```python
from build123d import *

# Parameters (mm, degrees)
SKETCH1_W                 = 180
SKETCH1_H                 = 100
BOSS_EXTRUDE1_DEPTH       = 60
F_3_0MM_DOWEL_HOLE1_D     = 5.25
F_3_0MM_DOWEL_HOLE1_DEPTH = 50
F_3_0MM_DOWEL_HOLE1_TIP   = 1.577259125
SHELL2_START              = 3
SHELL2_DEPTH              = 57
SHELL2_2_DEPTH            = 5.302681665
FILLET1_R                 = 5
FILLET2_R                 = 3
SKETCH4_R                 = 5.959707521
SKETCH4_W                 = 8
SKETCH4_H                 = 15
CUT_EXTRUDE1_DEPTH        = 10
SKETCH6_R                 = 5.5
CUT_EXTRUDE2_DEPTH        = 10
SKETCH9_R                 = 3.5
SKETCH9_R_2               = 5
SKETCH9_R_3               = 4
CUT_EXTRUDE3_DEPTH        = 7
SKETCH10_R                = 4
CUT_EXTRUDE4_DEPTH        = 10


with BuildPart() as part:
    # Sketch1 → Boss-Extrude1 (new body)
    with BuildSketch(Plane(origin=(0, 0, 0), x_dir=(1, 0, 0), z_dir=(0, 1, 0))):
        with Locations((90, -50)):
            Rectangle(SKETCH1_W, SKETCH1_H)
    extrude(amount=BOSS_EXTRUDE1_DEPTH)

    # Ø3.0mm Dowel Hole1
    with Locations(Plane(origin=(0, 60, 0), x_dir=(1, 0, 0), z_dir=(0, 1, 0))):
        with Locations((5.625, -5.625), (174.375, -5.625), (5.625, -94.375), (174.375, -94.375)):
            Hole(F_3_0MM_DOWEL_HOLE1_D / 2, depth=F_3_0MM_DOWEL_HOLE1_DEPTH)
            with Locations((0, 0, -(F_3_0MM_DOWEL_HOLE1_DEPTH + F_3_0MM_DOWEL_HOLE1_TIP / 2))):  # 118° drill point
                Cone(0, F_3_0MM_DOWEL_HOLE1_D / 2, F_3_0MM_DOWEL_HOLE1_TIP, mode=Mode.SUBTRACT)

    # Shell2: read off the stored shape, not the designer's step
    # Shell2 outline → Shell2 (cut)
    with BuildSketch(Plane(origin=(0, 0, 0), x_dir=(1, 0, 0), z_dir=(0, 1, 0)).offset(SHELL2_START)):
        with BuildLine():
            Line((169.400062814, -3), (10.599937186, -3))
            ThreePointArc((10.599937186, -3), (9.602475644, -9.602475644), (3, -10.599937186))
            Line((3, -10.599937186), (3, -89.400062814))
            ThreePointArc((3, -89.400062814), (9.602475644, -90.397524356), (10.599937186, -97))
            Line((10.599937186, -97), (169.400062814, -97))
            ThreePointArc((169.400062814, -97), (170.397524356, -90.397524356), (177, -89.400062814))
            Line((177, -89.400062814), (177, -10.599937186))
            ThreePointArc((177, -10.599937186), (170.397524356, -9.602475644), (169.400062814, -3))
        make_face()
    extrude(amount=SHELL2_DEPTH, mode=Mode.SUBTRACT)

    # Shell2 2 outline → Shell2 2 (cut)
    with BuildSketch(Plane(origin=(0, 0, 0), x_dir=(1, 0, 0), z_dir=(0, 1, 0)).offset(SHELL2_START)):
        with BuildLine():
            Line((10.599937186, -3), (3, -3))
            Line((3, -3), (3, -10.599937186))
            ThreePointArc((3, -10.599937186), (9.602475644, -9.602475644), (10.599937186, -3))
        make_face()
        with BuildLine():
            Line((177, -3), (169.400062814, -3))
            ThreePointArc((169.400062814, -3), (170.397524356, -9.602475644), (177, -10.599937186))
            Line((177, -10.599937186), (177, -3))
        make_face()
        with BuildLine():
            ThreePointArc((10.599937186, -97), (9.602475644, -90.397524356), (3, -89.400062814))
            Line((3, -89.400062814), (3, -97))
            Line((3, -97), (10.599937186, -97))
        make_face()
        with BuildLine():
            Line((177, -97), (177, -89.400062814))
            ThreePointArc((177, -89.400062814), (170.397524356, -90.397524356), (169.400062814, -97))
            Line((169.400062814, -97), (177, -97))
        make_face()
    extrude(amount=SHELL2_2_DEPTH, mode=Mode.SUBTRACT)

    # Shell2 3 outline → Shell2 3 (revolve)
    with BuildSketch(Plane(origin=(5.625, 0, 94.375), x_dir=(1, 0, 0), z_dir=(0, 0, 1))):
        Polygon((0, 8.302681673), (0, 4.922840683), (5.625000013, 8.302681673), align=None)
    revolve(axis=Axis((5.625, 0, 94.375), (0, 1, 0)))

    # Shell2 4 outline → Shell2 4 (revolve)
    with BuildSketch(Plane(origin=(174.375, 0, 94.375), x_dir=(1, 0, 0), z_dir=(0, 0, 1))):
        Polygon((0, 8.302681665), (0, 4.922840683), (5.625, 8.302681665), align=None)
    revolve(axis=Axis((174.375, 0, 94.375), (0, 1, 0)))

    # Shell2 5 outline → Shell2 5 (revolve)
    with BuildSketch(Plane(origin=(174.375, 0, 5.625), x_dir=(1, 0, 0), z_dir=(0, 0, 1))):
        Polygon((0, 8.302681673), (0, 4.922840683), (5.625000013, 8.302681673), align=None)
    revolve(axis=Axis((174.375, 0, 5.625), (0, 1, 0)))

    # Shell2 6 outline → Shell2 6 (revolve)
    with BuildSketch(Plane(origin=(5.625, 0, 5.625), x_dir=(1, 0, 0), z_dir=(0, 0, 1))):
        Polygon((0, 8.302681673), (0, 4.922840683), (5.625000013, 8.302681673), align=None)
    revolve(axis=Axis((5.625, 0, 5.625), (0, 1, 0)))

    # Fillet1
    fillet1_edges = [part.edges().sort_by_distance(p)[0] for p in [
        (0, 30, 0),
        (180, 30, 0),
        (180, 30, 100),
        (0, 30, 100),
    ]]
    fillet(fillet1_edges, radius=FILLET1_R)

    # Fillet2
    fillet2_edges = [part.edges().sort_by_distance(p)[0] for p in [
        (0, 0, 50),
        (90, 0, 0),
        (180, 0, 50),
        (90, 0, 100),
        (1.464466094, 0, 98.535533906),
        (178.535533906, 0, 98.535533906),
        (178.535533906, 0, 1.464466094),
        (1.464466094, 0, 1.464466094),
    ]]
    fillet(fillet2_edges, radius=FILLET2_R)

    # Sketch4 → Cut-Extrude1 (cut)
    with BuildSketch(Plane(origin=(180, 0, 0), x_dir=(0, 0, -1), z_dir=(1, 0, 0))):
        with Locations((-24, 45)):
            Circle(SKETCH4_R)
        with Locations((-24, 27.5)):
            Rectangle(SKETCH4_W, SKETCH4_H)
    extrude(amount=-CUT_EXTRUDE1_DEPTH, mode=Mode.SUBTRACT)

    # Sketch6 → Cut-Extrude2 (cut)
    with BuildSketch(Plane.XZ):
        with Locations(Location((25.5, 82, 0), (0, 0, 270))):
            Circle(SKETCH6_R)
        with Locations(Location((48, 82, 0), (0, 0, 270))):
            Circle(SKETCH6_R)
    extrude(amount=-CUT_EXTRUDE2_DEPTH, mode=Mode.SUBTRACT)

    # Sketch9 → Cut-Extrude3 (cut)
    with BuildSketch(Plane.XZ):
        with Locations(Location((21, 23, 0), (0, 0, 270))):
            Circle(SKETCH9_R)
        with Locations(Location((58, 23, 0), (0, 0, 270))):
            Circle(SKETCH9_R)
        with Locations(Location((95, 23, 0), (0, 0, 270))):
            Circle(SKETCH9_R)
        with Locations(Location((21, 52.813509344, 0), (0, 0, 270))):
            Circle(SKETCH9_R_2)
        with Locations(Location((58, 52.813509344, 0), (0, 0, 270))):
            Circle(SKETCH9_R)
        with Locations(Location((95, 52.813509344, 0), (0, 0, 270))):
            Circle(SKETCH9_R_3)
    extrude(amount=-CUT_EXTRUDE3_DEPTH, mode=Mode.SUBTRACT)

    # Sketch10 → Cut-Extrude4 (cut)
    with BuildSketch(Plane.XZ):
        with Locations(Location((76.5, 81.714376639, 0), (0, 0, 270))):
            Circle(SKETCH10_R)
    extrude(amount=-CUT_EXTRUDE4_DEPTH, mode=Mode.SUBTRACT)


solid = part.part
```
Geometry check sheet. Reference: the model listing, model coordinates, mm. A direction names the side the tool comes from. Give positions to 0.01 mm unless a question says otherwise; leave off trailing zeros. Loops run counter-clockwise (first coordinate to the right, second up) from the corner with the lowest first, then second, coordinate; pieces in that order, holes last. Notation, with made-up numbers: M -1.5,25.25 L 49.5,25.25 A29 cw 49.5,47.25 Z; hole C 22.25,45 d9. An arc over 180 degrees is marked long. Write item = value, one per line. Start each with the question number.
1. Section check C-C, the plane y = 31. Enter the section's corners in (x, z) (3 decimals), plus the area to 3 significant figures.
2. Draft check along Z on faces 4 (the face through (5.526, 8.697, 94.82)), 5 (the face through (89, 0, 49)), 6 (the face through (178, 32, 99)), 7 (the face through (1, 32, 2)). Enter one of: +Z half, -Z half, draft (parallel to the pull), parting line (faces both ways), or undercut.
3. Section check D-D, the plane x = 128. Enter the section's corners in (y, z).
4. Go/stop test with flat-tipped pins: P1, Ø6.5, axis at x = 76.5, z = 81.71, coming from the +Y side; P2, Ø0.9, axis at x = 178.5, y = 28, coming from the -Z side; P3, Ø4, axis at x = 174.375, z = 5.625, coming from the +Y side; P4, Ø10, axis at x = 37.5, z = 73, coming from the -Y side. Record where each tip stops, or that it passes through.
5. Section check A-A, the plane x = 95. Enter the section's corners in (y, z), plus the area to 3 significant figures.
6. Thickness scan on probe 1 along X at (y, z) = (58, 94); probe 2 along X at (y, z) = (26, 75.5); probe 3 along Z at (x, y) = (59.5, 49). Record the ranges inside material, lowest first.
7. Section check B-B, the plane z = 54. Enter the section's corners in (x, y), plus the area to 3 significant figures.
8. Tool access check on faces 1 (the face through (6.08, 5.51, 6.49)), 2 (the face through (23.95, 1.48, 21.12)), 3 (the face through (6.19, 34.65, 96.94)). Record the directions out of +Z, -Z, +X, -X, +Y, -Y that give a thin tool (end or side, any length) a straight path to the whole face; none if there is none.
Values follow:
q1.outline = M 0,5 A5 ccw 5,0 L 175,0 A5 ccw 180,5 L 180,20 L 177,20 L 177,10.6 A5.625 ccw 169.4,3 L 10.6,3 A5.625 ccw 3,10.6 L 3,89.4 A5.625 ccw 10.6,97 L 169.4,97 A5.625 ccw 177,89.4 L 177,28 L 180,28 L 180,95 A5 ccw 175,100 L 5,100 A5 ccw 0,95 Z; hole C 5.625,5.625 d5.25; hole C 5.625,94.375 d5.25; hole C 174.375,5.625 d5.25; hole C 174.375,94.375 d5.25
q1.area = 1,750 mm^2
q2.face_4 = undercut
q2.face_5 = draft
q2.face_6 = +Z half
q2.face_7 = -Z half
q3.outline = M 0,3 A3 ccw 3,0 L 60,0 L 60,3 L 3,3 L 3,97 L 60,97 L 60,100 L 3,100 A3 ccw 0,97 Z
q4.P1 = through
q4.P2 = 1.04
q4.P3 = 9.62
q4.P4 = 0
q5.outline = M 0,3 A3 ccw 3,0 L 60,0 L 60,3 L 3,3 L 3,19.5 L 0,19.5 Z; M 0,26.5 L 3,26.5 L 3,48.81 L 0,48.81 Z; M 0,56.81 L 3,56.81 L 3,97 L 60,97 L 60,100 L 3,100 A3 ccw 0,97 Z
q5.area = 593 mm^2
q6.probe_1 = 0 to 3.03, 8.22 to 11.24, 168.76 to 171.78, 176.97 to 180
q6.probe_2 = 0 to 3, 177 to 180
q6.probe_3 = 0 to 3, 97 to 100
q7.outline = M 0,3 A3 ccw 3,0 L 16.14,0 L 16.14,3 L 3,3 L 3,60 L 0,60 Z; M 25.86,0 L 54.71,0 L 54.71,3 L 25.86,3 Z; M 61.29,0 L 91.18,0 L 91.18,3 L 61.29,3 Z; M 98.82,0 L 177,0 A3 ccw 180,3 L 180,60 L 177,60 L 177,3 L 98.82,3 Z
q7.area = 806 mm^2
q8.face_1 = none
q8.face_2 = +Y, -Y
q8.face_3 = +Y
